from build123d import *

# Parameters (mm, degrees)
SKETCH1_W            = 60
SKETCH1_H            = 90
BOSS_EXTRUDE1_DEPTH  = 5
SKETCH2_W            = 5
SKETCH2_H            = 25
BOSS_EXTRUDE2_DEPTH  = 3
SKETCH3_R            = 14
SKETCH3_R_2          = 9
SKETCH3_R_3          = 4.5
SKETCH3_R_4          = 4
SKETCH3_R_5          = 2.5
CUT_EXTRUDE1_DEPTH   = 57.026779311
SKETCH4_R            = 1.75
CUT_EXTRUDE2_DEPTH   = 57.026779311
FILLET1_R            = 1.5
FILLET2_R            = 1.5
BOSS_EXTRUDE3_DEPTH  = 3.5
SKETCH6_R            = 1.25
CUT_EXTRUDE3_DEPTH   = 57.446877835
FILLET3_R            = 5
FILLET3_OF_MIRROR2_R = 5
SKETCH12_R           = 1.5
CUT_EXTRUDE7_DEPTH   = 57.44687782
BOSS_EXTRUDE5_DEPTH  = 8
FILLET5_R            = 3
SKETCH15_R           = 1.5
CUT_EXTRUDE8_DEPTH   = 5
FILLET5_OF_MIRROR3_R = 3


# Some blends are built 0.0001 mm under size
with BuildPart() as part:
    # Sketch1 → Boss-Extrude1 (new body)
    with BuildSketch(Plane.XY):
        Rectangle(SKETCH1_W, SKETCH1_H)
    extrude(amount=BOSS_EXTRUDE1_DEPTH)

    # Sketch2 → Boss-Extrude2 (add)
    with BuildSketch(Plane(origin=(30, 0, 0), x_dir=(0, 0, -1), z_dir=(1, 0, 0))):
        with Locations((-2.5, -32.5)):
            Rectangle(SKETCH2_W, SKETCH2_H)
    boss_extrude2 = extrude(amount=BOSS_EXTRUDE2_DEPTH)

    # Mirror1: Boss-Extrude2 across plane
    add(boss_extrude2.mirror(Plane(origin=(0, 0, 0), x_dir=(0, 0, 1), z_dir=(1, 0, 0))))

    # Sketch3 → Cut-Extrude1 (cut, through all)
    with BuildSketch(Plane.XY.offset(5)):
        with Locations((0, -23)):
            Circle(SKETCH3_R)
        with Locations((0, 23)):
            Circle(SKETCH3_R)
        with Locations((15, 0)):
            Circle(SKETCH3_R_2)
        with Locations((-15, 0)):
            Circle(SKETCH3_R_2)
        with Locations((-22.5, -16)):
            Circle(SKETCH3_R_3)
        with Locations((-18, -39)):
            Circle(SKETCH3_R_4)
        with Locations((22.5, -16)):
            Circle(SKETCH3_R_3)
        with Locations((18, -39)):
            Circle(SKETCH3_R_4)
        with Locations((22.5, 16)):
            Circle(SKETCH3_R_3)
        with Locations((22.5, 30)):
            Circle(SKETCH3_R_3)
        with Locations((-22.5, 30)):
            Circle(SKETCH3_R_3)
        with Locations((-22.5, 16)):
            Circle(SKETCH3_R_3)
        Circle(SKETCH3_R_5)
        with BuildLine():
            Line((30, -10), (30, 10))
            ThreePointArc((30, 10), (29.192459912, 7.084524053), (27, 5))
            ThreePointArc((27, 5), (28, 0), (27, -5))
            ThreePointArc((27, -5), (29.192459912, -7.084524053), (30, -10))
        make_face()
        with BuildLine():
            Line((30, 18), (30, 28))
            ThreePointArc((30, 28), (29.192459912, 25.084524053), (27, 23))
            ThreePointArc((27, 23), (29.192459912, 20.915475947), (30, 18))
        make_face()
        with BuildLine():
            Line((-30, 18), (-30, 28))
            ThreePointArc((-30, 28), (-29.192459912, 25.084524053), (-27, 23))
            ThreePointArc((-27, 23), (-29.192459912, 20.915475947), (-30, 18))
        make_face()
        with BuildLine():
            Line((-30, -10), (-30, 10))
            ThreePointArc((-30, 10), (-29.192459912, 7.084524053), (-27, 5))
            ThreePointArc((-27, 5), (-28, 0), (-27, -5))
            ThreePointArc((-27, -5), (-29.192459912, -7.084524053), (-30, -10))
        make_face()
    extrude(amount=-CUT_EXTRUDE1_DEPTH, mode=Mode.SUBTRACT)

    # Sketch4 → Cut-Extrude2 (cut, through all)
    with BuildSketch(Plane.XY.offset(5)):
        with Locations((-30, -37)):
            Circle(SKETCH4_R)
        with Locations((30, -37)):
            Circle(SKETCH4_R)
    extrude(amount=-CUT_EXTRUDE2_DEPTH, mode=Mode.SUBTRACT)

    # Fillet1
    fillet1_edges = [part.edges().sort_by_distance(p)[0] for p in [
        (-33, -20, 2.5),
        (-33, -45, 2.5),
        (-30, -20, 2.5),
        (33, -45, 2.5),
        (33, -20, 2.5),
        (30, -20, 2.5),
    ]]
    fillet(fillet1_edges, radius=FILLET1_R - 0.0001)  # a hair under: the kernel refuses the full size

    # Fillet2
    fillet2_edges = [part.edges().sort_by_distance(p)[0] for p in [
        (27, -5, 2.5),
        (27, 5, 2.5),
        (27, 23, 2.5),
        (-27, 23, 2.5),
        (-27, -5, 2.5),
        (-27, 5, 2.5),
    ]]
    fillet(fillet2_edges, radius=FILLET2_R)

    # Sketch5 → Boss-Extrude3 (add)
    with BuildSketch(Plane.XY.offset(5)):
        with BuildLine():
            Line((24, 45), (30, 45))
            Line((30, 45), (30, 39.5))
            Line((30, 39.5), (27, 39.5))
            ThreePointArc((27, 39.5), (24.878679656, 40.378679656), (24, 42.5))
            Line((24, 42.5), (24, 45))
        make_face()
    boss_extrude3 = extrude(amount=BOSS_EXTRUDE3_DEPTH)

    # Sketch6 → Cut-Extrude3 (cut, through all)
    with BuildSketch(Plane.XY.offset(8.5)):
        with Locations((27, 42.5)):
            Circle(SKETCH6_R)
    cut_extrude3 = extrude(amount=-CUT_EXTRUDE3_DEPTH, mode=Mode.SUBTRACT)

    # Fillet3
    # the kernel refuses this fillet: 5 mm, written as the material it adds along each edge
    with BuildSketch(Plane(origin=(24, 42.5, 5), x_dir=(-1, 0, 0), z_dir=(0, 1, 0))) as fillet3_piece_1:
        with BuildLine():
            CenterArc((4.769696007, 5), FILLET3_R, 197.457603124, 72.542396876)
            Line((0, 3.5), (-0.09539392, 3.47))
            ThreePointArc((-0.09539392, 3.47), (-0.1, 1.75), (-0.1, 0))
            Line((-0.1, 0), (0, -0.1))
            Line((0, -0.1), (4.769696007, -0.1))
            Line((4.769696007, -0.1), (4.769696007, 0))
        make_face()
    extrude(amount=2.5)
    with BuildSketch(Plane(origin=(27, 42.5, 5), x_dir=(0, -1, 0), z_dir=(1, 0, 0))) as fillet3_piece_2:
        with BuildLine():
            CenterArc((7.769696007, -5), FILLET3_R, 90, 72.542396876)
            Line((3, -3.5), (2.90460608, -3.47))
            ThreePointArc((2.90460608, -3.47), (2.9, -1.75), (2.9, 0))
            Line((2.9, 0), (3, 0.1))
            Line((3, 0.1), (7.769696007, 0.1))
            Line((7.769696007, 0.1), (7.769696007, 0))
        make_face()
    revolve(axis=Axis((27, 42.5, 5), (0, 0, -1)), revolution_arc=90)
    with BuildSketch(Plane(origin=(30, 39.5, 5), x_dir=(0, -1, 0), z_dir=(-1, 0, 0))) as fillet3_piece_3:
        with BuildLine():
            CenterArc((4.769696007, 5), FILLET3_R, 197.457603124, 72.542396876)
            Line((0, 3.5), (-0.09539392, 3.47))
            ThreePointArc((-0.09539392, 3.47), (-0.1, 1.75), (-0.1, 0))
            Line((-0.1, 0), (0, -0.1))
            Line((0, -0.1), (4.769696007, -0.1))
            Line((4.769696007, -0.1), (4.769696007, 0))
        make_face()
    extrude(amount=3)

    # Mirror2: Boss-Extrude3, Cut-Extrude3 across plane
    add(boss_extrude3.mirror(Plane(origin=(0, 0, 0), x_dir=(0, 0, 1), z_dir=(1, 0, 0))))
    add(cut_extrude3.mirror(Plane(origin=(0, 0, 0), x_dir=(0, 0, 1), z_dir=(1, 0, 0))), mode=Mode.SUBTRACT)

    # Fillet3 of Mirror2
    # the kernel refuses this fillet: 5 mm, written as the material it adds along each edge
    with BuildSketch(Plane(origin=(-24, 42.5, 5), x_dir=(1, 0, 0), z_dir=(0, 1, 0))) as fillet3_of_mirror2_piece_1:
        with BuildLine():
            CenterArc((4.769696007, -5), FILLET3_OF_MIRROR2_R, 90, 72.542396876)
            Line((0, -3.5), (-0.09539392, -3.47))
            ThreePointArc((-0.09539392, -3.47), (-0.1, -1.75), (-0.1, 0))
            Line((-0.1, 0), (0, 0.1))
            Line((0, 0.1), (4.769696007, 0.1))
            Line((4.769696007, 0.1), (4.769696007, 0))
        make_face()
    extrude(amount=2.5)
    with BuildSketch(Plane(origin=(-27, 42.5, 5), x_dir=(0, -1, 0), z_dir=(-1, 0, 0))) as fillet3_of_mirror2_piece_2:
        with BuildLine():
            CenterArc((7.769696007, 5), FILLET3_OF_MIRROR2_R, 197.457603124, 72.542396876)
            Line((3, 3.5), (2.90460608, 3.47))
            ThreePointArc((2.90460608, 3.47), (2.9, 1.75), (2.9, 0))
            Line((2.9, 0), (3, -0.1))
            Line((3, -0.1), (7.769696007, -0.1))
            Line((7.769696007, -0.1), (7.769696007, 0))
        make_face()
    revolve(axis=Axis((-27, 42.5, 5), (0, 0, 1)), revolution_arc=90)
    with BuildSketch(Plane(origin=(-30, 39.5, 5), x_dir=(0, -1, 0), z_dir=(1, 0, 0))) as fillet3_of_mirror2_piece_3:
        with BuildLine():
            CenterArc((4.769696007, -5), FILLET3_OF_MIRROR2_R, 90, 72.542396876)
            Line((0, -3.5), (-0.09539392, -3.47))
            ThreePointArc((-0.09539392, -3.47), (-0.1, -1.75), (-0.1, 0))
            Line((-0.1, 0), (0, 0.1))
            Line((0, 0.1), (4.769696007, 0.1))
            Line((4.769696007, 0.1), (4.769696007, 0))
        make_face()
    extrude(amount=3)

    # Sketch12 → Cut-Extrude7 (cut, through all)
    with BuildSketch(Plane(origin=(0, 0, 0), x_dir=(-1, 0, 0), z_dir=(0, 0, -1))):
        with Locations((-13.5, 35.369741957)):
            Circle(SKETCH12_R)
        with Locations((0, 41)):
            Circle(SKETCH12_R)
        with Locations((13.5, 35.369741957)):
            Circle(SKETCH12_R)
    extrude(amount=-CUT_EXTRUDE7_DEPTH, mode=Mode.SUBTRACT)

    # Sketch14 → Boss-Extrude5 (add)
    with BuildSketch(Plane(origin=(33, 0, 0), x_dir=(0, 0, -1), z_dir=(1, 0, 0))):
        with BuildLine():
            Line((-5, -24), (-5, -32))
            ThreePointArc((-5, -32), (-9, -28), (-5, -24))
        make_face()
    boss_extrude5 = extrude(amount=-BOSS_EXTRUDE5_DEPTH)

    # Fillet5
    fillet5_edges = [part.edges().sort_by_distance(p)[0] for p in [
        (29, -32, 5),
        (29, -24, 5),
    ]]
    fillet(fillet5_edges, radius=FILLET5_R)

    # Sketch15 → Cut-Extrude8 (cut)
    with BuildSketch(Plane(origin=(33, 0, 0), x_dir=(0, 0, -1), z_dir=(1, 0, 0))):
        with Locations((-5, -28)):
            Circle(SKETCH15_R)
    cut_extrude8 = extrude(amount=-CUT_EXTRUDE8_DEPTH, mode=Mode.SUBTRACT)

    # Mirror3: Boss-Extrude5, Cut-Extrude8 across plane
    add(boss_extrude5.mirror(Plane(origin=(0, 0, 0), x_dir=(0, 0, 1), z_dir=(1, 0, 0))))
    add(cut_extrude8.mirror(Plane(origin=(0, 0, 0), x_dir=(0, 0, 1), z_dir=(1, 0, 0))), mode=Mode.SUBTRACT)

    # Fillet5 of Mirror3
    fillet5_of_mirror3_edges = [part.edges().sort_by_distance(p)[0] for p in [
        (-29, -32, 5),
        (-29, -24, 5),
    ]]
    fillet(fillet5_of_mirror3_edges, radius=FILLET5_OF_MIRROR3_R)


solid = part.part
Geometry: final body of the model. Coordinates: model frame, mm. A direction names the side the tool comes from. Give positions to 0.01 mm unless a question says otherwise; leave off trailing zeros. Loops run counter-clockwise (first coordinate to the right, second up) from the corner with the lowest first, then second, coordinate; pieces in that order, holes last. Notation, with made-up numbers: (-0.75, 51.25) -> (23.25, 51.25) arc R26 ccw to (23.25, 74.25) -> close; hole circle Ø7 at (-0.75, -17). An arc over 180 degrees is marked (long way). Put each result on its own line as item: value.
1. Cut plane D-D (x = -20.5). Count the separate pieces of the cut face and the enclosed holes in it, plus the area to 3 significant figures.
Taken from the geometry:
separate pieces: 6
enclosed holes: 0
area: 227 mm2
2. Pull-direction query (X, two-part tool) for faces 1 (the cylindrical face through (-28.944, -23.259, 5.452)), 2 (the cylindrical face through (-29.457, 7.579, 2.535)), 3 (the flat face through (25, -28, 7)); classes: released by +X, released by -X, zero draft, split by the parting line, or undercut.
Taken from the geometry:
face 1: zero draft
face 2: released by -X
face 3: undercut
3. Ray query, line 1 along Y through (x, z) = (22.5, 2); line 2 along Y through (x, z) = (-10, 1.75); line 3 along X through (y, z) = (-19.5, 4). Return the intervals inside material, ascending. Write a range as [from, to].
Taken from the geometry:
line 1: y = [-45, -20.5], [-11.5, -4.97], [4.97, 11.5], [20.5, 25.5], [34.5, 45]
line 2: y = [-45, -32.8], [-13.2, -7.48], [7.48, 13.2], [32.8, 45]
line 3: x = [-30.38, -25.33], [-19.67, -13.56], [13.56, 19.67], [25.33, 30.38]
4. Cut plane B-B (y = -7.5). Return the cut outline in (x, z).
Taken from the geometry:
outline: (-29.42, 0) -> (-19.97, 0) -> (-19.97, 5) -> (-29.42, 5) -> close; (-10.03, 0) -> (10.03, 0) -> (10.03, 5) -> (-10.03, 5) -> close; (19.97, 0) -> (29.42, 0) -> (29.42, 5) -> (19.97, 5) -> close
5. Pin query (flat end, axial travel): P1, Ø7, axis at x = 18, y = -39, coming from the +Z side; P2, Ø5, axis at x = 0, y = 41, coming from the -Z side; P3, Ø2, axis at x = 25, z = 8, coming from the -Y side; P4, Ø1.5, axis at y = 14, z = 2.5, coming from the +X side. Return the tip coordinate at first contact, or that it passes through.
Taken from the geometry:
P1: passes through
P2: stops at z = 0
P3: stops at y = -31.46
P4: stops at x = 30
6. Cut plane C-C (y = -23). Return the cut outline in (x, z), plus the area to 3 significant figures.
Taken from the geometry:
outline: (-33, 0) -> (-14, 0) -> (-14, 5) -> (-25, 5) -> (-25, 5.31) -> (-33, 5.31) -> close; (14, 0) -> (33, 0) -> (33, 5.31) -> (25, 5.31) -> (25, 5) -> (14, 5) -> close
area: 195 mm2
7. Set-up query: faces 4 (the cylindrical face through (28.521, 37.724, 5.995)), 5 (the cylindrical face through (29.43, -7.52, 2.54)), 6 (the flat face through (-28.4, 42.3, 8.5)), 7 (the flat face through (30, -14, 2)). Return all of +Z, -Z, +X, -X, +Y, -Y with unobstructed straight access to the full face (end or side cutting, diameter ignored); none if empty.
Taken from the geometry:
face 4: +Z, +X, -X
face 5: +Z, -Z, +X
face 6: +Z, +X, -X, +Y
face 7: +Z, -Z, +X, +Y
8. Cut plane A-A (y = 17). Return the cut outline in (x, z), plus the area to 3 significant figures.
Taken from the geometry:
outline: (-30, 0) -> (-26.89, 0) -> (-26.89, 5) -> (-30, 5) -> close; (-18.11, 0) -> (-12.65, 0) -> (-12.65, 5) -> (-18.11, 5) -> close; (12.65, 0) -> (18.11, 0) -> (18.11, 5) -> (12.65, 5) -> close; (26.89, 0) -> (30, 0) -> (30, 5) -> (26.89, 5) -> close
area: 85.8 mm2
